Could you check a few things on this model? Use its own coordinates, in mm. A direction names the side the tool comes from. Round coordinates to 2 decimals unless told otherwise and drop trailing zeros. Loops run counter-clockwise (first coordinate to the right, second up) from the corner with the lowest first, then second, coordinate; pieces in that order, holes last.
from build123d import *

# Parameters (mm, degrees)
SKETCH_1_W           = 20
SKETCH_1_H           = 20
EXTRUDE_1_DEPTH      = 4
SKETCH_2_W           = 12.9
SKETCH_2_H           = 20
EXTRUDE_2_DEPTH      = 3.8
SKETCH_3_R           = 1.6
CUT_EXTRUDE_1_DEPTH  = 30.340074983
SKETCH_4_W           = 5.8
SKETCH_4_H           = 20
SKETCH_4_R           = 1.6
EXTRUDE_3_DEPTH      = 1.5
SKETCH_5_R           = 3
CUT_EXTRUDE_3_DEPTH  = 2.4
SKETCH_6_W           = 20
SKETCH_6_H           = 4
EXTRUDE_4_DEPTH      = 3
EXTRUDE_START        = 4
SKETCH_7_W           = 23
SKETCH_7_H           = 20
SKETCH_7_R           = 3
EXTRUDE_5_DEPTH      = 4
SKETCH_9_W           = 10.1
SKETCH_9_H           = 20
EXTRUDE_6_DEPTH      = 2
EXTRUDE_7_DEPTH      = 5
CHAMFER_7_SIZE       = 10
CHAMFER_7_SIZE2      = 5.773502692
CHAMFER_8_SIZE       = 5
CHAMFER_9_SIZE       = 8
CHAMFER_9_SIZE2      = 4.618802154
CUT_EXTRUDE_9_DEPTH  = 10.1
CUT_EXTRUDE_10_REACH = 38.481
CHAMFER_10_SIZE      = 1.5
CHAMFER_11_SIZE      = 0.4
EXTRUDE_8_DEPTH      = 1.8
EXTRUDE_10_DEPTH     = 10.1


with BuildPart() as part:
    # 草图1 → 凸台-拉伸1 (new body)
    with BuildSketch(Plane(origin=(0, 0, 0), x_dir=(1, 0, 0), z_dir=(0, 1, 0))):
        with Locations((10, 10)):
            Rectangle(SKETCH_1_W, SKETCH_1_H)
    extrude(amount=EXTRUDE_1_DEPTH)

    # 草图2 → 凸台-拉伸2 (add)
    with BuildSketch(Plane(origin=(0, 4, 0), x_dir=(1, 0, 0), z_dir=(0, 1, 0))):
        with Locations((6.45, 10)):
            Rectangle(SKETCH_2_W, SKETCH_2_H)
    extrude(amount=EXTRUDE_2_DEPTH)

    # 草图3 → 切除-拉伸1 (cut, through all)
    with BuildSketch(Plane(origin=(0, 0, 0), x_dir=(-1, 0, 0), z_dir=(0, -1, 0))):
        with Locations(Location((-10, 5, 0), (0, 0, 90))):
            Circle(SKETCH_3_R)
        with Locations(Location((-10, 13, 0), (0, 0, 90))):
            Circle(SKETCH_3_R)
    extrude(amount=-CUT_EXTRUDE_1_DEPTH, mode=Mode.SUBTRACT)

    # 草图4 → 凸台-拉伸3 (add)
    with BuildSketch(Plane(origin=(0, 7.8, 0), x_dir=(1, 0, 0), z_dir=(0, 1, 0))):
        with Locations((10, 10)):
            Rectangle(SKETCH_4_W, SKETCH_4_H)
        with Locations(Location((10, 13, 0), (0, 0, 90))):
            Circle(SKETCH_4_R, mode=Mode.SUBTRACT)
        with Locations(Location((10, 5, 0), (0, 0, 90))):
            Circle(SKETCH_4_R, mode=Mode.SUBTRACT)
    extrude(amount=EXTRUDE_3_DEPTH)

    # 草图5 → 切除-拉伸3 (cut)
    with BuildSketch(Plane(origin=(0, 0, 0), x_dir=(-1, 0, 0), z_dir=(0, -1, 0))):
        with Locations(Location((-10, 5, 0), (0, 0, 90))):
            Circle(SKETCH_5_R)
        with Locations(Location((-10, 13, 0), (0, 0, 90))):
            Circle(SKETCH_5_R)
    extrude(amount=-CUT_EXTRUDE_3_DEPTH, mode=Mode.SUBTRACT)

    # 草图6 → 凸台-拉伸4 (add)
    with BuildSketch(Plane(origin=(20, 0, 0), x_dir=(0, 0, -1), z_dir=(1, 0, 0))):
        with Locations((10, 2)):
            Rectangle(SKETCH_6_W, SKETCH_6_H)
    extrude(amount=EXTRUDE_4_DEPTH)

    # 草图7 → 凸台-拉伸5 (add)
    with BuildSketch(Plane(origin=(0, 0, 0), x_dir=(-1, 0, 0), z_dir=(0, -1, 0)).offset(EXTRUDE_START)):
        with Locations((-11.5, 10)):
            Rectangle(SKETCH_7_W, SKETCH_7_H)
        with Locations(Location((-10, 13, 0), (0, 0, 90))):
            Circle(SKETCH_7_R, mode=Mode.SUBTRACT)
        with Locations(Location((-10, 5, 0), (0, 0, 90))):
            Circle(SKETCH_7_R, mode=Mode.SUBTRACT)
    extrude(amount=-EXTRUDE_5_DEPTH)

    # 草图9 → 凸台-拉伸6 (add)
    with BuildSketch(Plane(origin=(0, 4, 0), x_dir=(1, 0, 0), z_dir=(0, 1, 0))):
        with Locations((17.95, 10)):
            Rectangle(SKETCH_9_W, SKETCH_9_H)
    extrude(amount=EXTRUDE_6_DEPTH)

    # 草图11 → 凸台-拉伸7 (add)
    with BuildSketch(Plane(origin=(0, 0, -20), x_dir=(-1, 0, 0), z_dir=(0, 0, -1))):
        Polygon((-23, 6), (-23, -4), (0, -4), (0, 7.8), (-7.1, 7.8), (-7.1, 9.3), (-12.9, 9.3), (-12.9, 6), align=None)
    extrude(amount=EXTRUDE_7_DEPTH)

    # 倒角7
    chamfer_7_edges = [part.edges().sort_by_distance(p)[0] for p in [
        (0, -4, -12.5),
    ]]
    chamfer_7_side = [part.faces().sort_by_distance(p)[0] for p in [
        (0, 1.9, -12.5),
    ]]
    chamfer(chamfer_7_edges, length=CHAMFER_7_SIZE, length2=CHAMFER_7_SIZE2, reference=chamfer_7_side[0])

    # 倒角8
    chamfer_8_edges = [part.edges().sort_by_distance(p)[0] for p in [
        (23, 1, 0),
    ]]
    chamfer(chamfer_8_edges, length=CHAMFER_8_SIZE)

    # 倒角9
    chamfer_9_edges = [part.edges().sort_by_distance(p)[0] for p in [
        (20.5, -4, -2.5),
    ]]
    chamfer_9_side = [part.faces().sort_by_distance(p)[0] for p in [
        (20.5, 1, -2.5),
    ]]
    chamfer(chamfer_9_edges, length=CHAMFER_9_SIZE, length2=CHAMFER_9_SIZE2, reference=chamfer_9_side[0])

    # 草图15 → 切除-拉伸9 (cut)
    with BuildSketch(Plane(origin=(23, 0, 0), x_dir=(0, 0, -1), z_dir=(1, 0, 0))):
        Polygon((25, -3), (25, 6), (7, 6), align=None)
    extrude(amount=-CUT_EXTRUDE_9_DEPTH, mode=Mode.SUBTRACT)

    # 切除-拉伸10: up to this plane
    cut_extrude_10_end = Plane(origin=(-7.224611797, 6, -7), z_dir=(0, -0.894427190999916, 0.447213595499958))
    # 草图16 → 切除-拉伸10 (cut, up to the surface)
    with BuildSketch(Plane(origin=(0, 9.3, 0), x_dir=(1, 0, 0), z_dir=(0, 1, 0)), mode=Mode.PRIVATE) as cut_extrude_10_sk1:
        Polygon((7.9, 25), (12.9, 25), (12.9, 14), align=None)
    cut_extrude_10_tool1 = split(extrude(cut_extrude_10_sk1.sketch, amount=-CUT_EXTRUDE_10_REACH, mode=Mode.PRIVATE), bisect_by=cut_extrude_10_end, keep=Keep.BOTH, mode=Mode.PRIVATE)
    add(cut_extrude_10_tool1.solids().sort_by_distance((11.233333, 9.3, -21.333333))[0], mode=Mode.SUBTRACT)

    # 倒角10
    # the kernel refuses this chamfer: 1.5 mm, written as the material it takes off along each edge
    with BuildSketch(Plane(origin=(10, 2.4, -13), x_dir=(0, 0, -1), z_dir=(-1, 0, 0))) as chamfer_10_piece_1_section:
        Polygon((1.6, -CHAMFER_10_SIZE), (1.6 + CHAMFER_10_SIZE, 0), (1.6, 0), align=None)
    chamfer_10_piece_1 = revolve(axis=Axis((10, 2.4, -13), (0, -1, 0)), mode=Mode.PRIVATE)
    chamfer_10_piece_1 = chamfer_10_piece_1 & Plane(origin=(10, 3.20338318, -13), x_dir=(0, 0, -1), z_dir=(0, -1, 0)) * Cylinder(3, 13, mode=Mode.PRIVATE)
    add(chamfer_10_piece_1, mode=Mode.SUBTRACT)
    with BuildSketch(Plane(origin=(10, 2.4, -5), x_dir=(0, 0, -1), z_dir=(-1, 0, 0))) as chamfer_10_piece_2_section:
        Polygon((1.6, -CHAMFER_10_SIZE), (1.6 + CHAMFER_10_SIZE, 0), (1.6, 0), align=None)
    chamfer_10_piece_2 = revolve(axis=Axis((10, 2.4, -5), (0, -1, 0)), mode=Mode.PRIVATE)
    chamfer_10_piece_2 = chamfer_10_piece_2 & Plane(origin=(10, 3.20338318, -5), x_dir=(0, 0, -1), z_dir=(0, -1, 0)) * Cylinder(3, 13, mode=Mode.PRIVATE)
    add(chamfer_10_piece_2, mode=Mode.SUBTRACT)

    # 倒角11
    # the kernel refuses this chamfer: 0.4 mm, written as the material it takes off along each edge
    with BuildSketch(Plane(origin=(13.325667997, 9.3, -13.063530407), x_dir=(-0.9100222832929536, 0.027495876610587288, 0.4136464924058883), z_dir=(-0.4138029443011842, 0, -0.9103664774626047))) as chamfer_11_piece_1:
        Polygon((CHAMFER_11_SIZE * 0.999621916911, -CHAMFER_11_SIZE * 0.0274958766106), (-CHAMFER_11_SIZE * 0.0274958766106, -CHAMFER_11_SIZE * 0.999621916911), (0, 0), align=None)
    extrude(amount=14.140392364, mode=Mode.SUBTRACT)
    with BuildSketch(Plane(origin=(12.9, 9.3, 1.028673195), x_dir=(-0.9996219169112966, 0.027495876610587302, 0), z_dir=(0, 0, -1))) as chamfer_11_piece_2:
        Polygon((CHAMFER_11_SIZE * 0.999621916911, -CHAMFER_11_SIZE * 0.0274958766106), (-CHAMFER_11_SIZE * 0.0274958766106, -CHAMFER_11_SIZE * 0.999621916911), (0, 0), align=None)
    extrude(amount=16.05734639, mode=Mode.SUBTRACT)
    with BuildSketch(Plane(origin=(7.1, 9.3, 1.028673195), x_dir=(0.9996219169112966, 0.027495876610587302, 0), z_dir=(0, 0, -1))) as chamfer_11_piece_3:
        Polygon((CHAMFER_11_SIZE * 0.999621916911, CHAMFER_11_SIZE * 0.0274958766106), (-CHAMFER_11_SIZE * 0.0274958766106, CHAMFER_11_SIZE * 0.999621916911), (0, 0), align=None)
    extrude(amount=27.05734639, mode=Mode.SUBTRACT)

    # 草图17 → 凸台-拉伸8 (add)
    with BuildSketch(Plane(origin=(0, 6, 0), x_dir=(1, 0, 0), z_dir=(0, 1, 0))):
        Polygon((23, 5), (23, 7), (12.9, 7), (12.9, 0), (18, 0), align=None)
    extrude(amount=EXTRUDE_8_DEPTH)

    # 草图19 → 凸台-拉伸10 (add)
    with BuildSketch(Plane(origin=(23, 0, 0), x_dir=(0, 0, -1), z_dir=(1, 0, 0))):
        Polygon((9.8, 7.8), (7, 7.8), (7, 6), (9.8, 4.6), align=None)
    extrude(amount=-EXTRUDE_10_DEPTH)


solid = part.part
Item 1: For faces 1 (the flat face through (7.1, 8, -12)), 2 (the flat face through (18, 7.8, -5)), 3 (the flat face through (9, 3, 0)), 4 (the cylindrical face through (10, -1, -2)), which set-ups out of +Z, -Z, +X, -X, +Y, -Y let a thin tool reach every point of the face, with its end or its side?
Results list:
face 1: +Z, -Z, -X, +Y
face 2: +Z, -Z, +X, +Y
face 3: +Z, +X, -X, +Y, -Y
face 4: -Y
Item 2: If we section it at A-A, the plane z = -13: Please give me the cut outline in (x, y), then the cut area to 3 significant figures.
Results list:
outline: (0, 6) - (5.77, -4) - (7, -4) - (7, 2.5) - (8.4, 3.9) - (8.4, 9.3) - (7.5, 9.3) - (7.1, 8.9) - (7.1, 7.8) - (0, 7.8) - close; (11.6, 3.9) - (13, 2.5) - (13, -4) - (23, -4) - (23, 3) - (12.9, 3) - (12.9, 8.9) - (12.5, 9.3) - (11.6, 9.3) - close
area: 140 mm2
Item 3: If we section it at D-D, the plane x = 13.75: Please give me the cut outline in (y, z), then the cut area to 3 significant figures.
Results list:
outline: (-4, -25) - (-3, -25) - (4.6, -9.8) - (7.8, -9.8) - (7.8, 0) - (-1.21, 0) - (-4, -2.28) - close
area: 185 mm2
Item 4: If I drill on line 1 along Z through (x, y) = (10.5, 1.5); line 2 along Z through (x, y) = (10, 6.75); line 3 along X through (y, z) = (5.9, -13), over which ranges is the centre line in solid material (lowest first)?
Results list:
line 1: z = -19.28 to -15.96, -10.04 to -7.96, -2.04 to 0
line 2: z = -20.38 to -14.6, -11.4 to -6.6, -3.4 to 0
line 3: x = 0.06 to 8.4, 11.6 to 12.9
Item 5: Will these pins go through, and if not, where does the flat tip stop? pin 1 (2.5 mm diameter, centred on x = 10, z = -5, fed in from +Y); pin 2 (3.5 mm diameter, centred on x = 2, z = -11, fed in from +Y); pin 3 (1.5 mm diameter, centred on x = 18.5, z = -12.5, fed in from +Y) (3 decimals); pin 4 (2.5 mm diameter, centred on x = 19.5, y = 5.5, fed in from -Z).
Results list:
pin 1: passes through
pin 2: stops at y = 7.8
pin 3: stops at y = 3.625
pin 4: stops at z = -10.5
Item 6: If we section it at C-C, the plane x = 10: Please give me the cut outline in (y, z), then the cut area to 3 significant figures.
Results list:
outline: (-4, -25) - (-3, -25) - (-0.69, -20.38) - (8.9, -20.38) - (9.3, -19.41) - (9.3, -14.6) - (3.9, -14.6) - (2.5, -16) - (-4, -16) - close; (-4, -10) - (2.5, -10) - (3.9, -11.4) - (9.3, -11.4) - (9.3, -6.6) - (3.9, -6.6) - (2.5, -8) - (-4, -8) - close; (-4, -2) - (2.5, -2) - (3.9, -3.4) - (9.3, -3.4) - (9.3, 0) - (-4, 0) - close
area: 155 mm2
Item 7: We'd pull the mould along Z, two halves only. Please class faces 5 (the flat face through (15, -4, -15)), 6 (the flat face through (20, 6, -2)), 7 (the cylindrical face through (10, -1, -10)), 8 (the flat face through (10.435, 4.356, -19.423)): released by +Z, released by -Z, zero draft, split by the parting line, or undercut.
Results list:
face 5: zero draft
face 6: released by +Z
face 7: undercut
face 8: released by -Z
Item 8: If we section it at B-B, the plane y = 7.25: Please give me the cut outline in (x, z).
Results list:
outline: (0, -25) - (7.9, -25) - (12.9, -14) - (12.9, -9.8) - (23, -9.8) - (23, -5) - (18, 0) - (0, 0) - close; hole circle Ø3.2 at (10, -13); hole circle Ø3.2 at (10, -5)
